Answer from the drawing. Dimensions are ordinates in mm from the lowest x, y and z of the part. A direction names the side the tool comes from. Coordinates: 2 decimals unless noted, no trailing zeros. Write each loop counter-clockwise with the first axis right and the second up, starting at its lowest first coordinate (ties: lowest second). Pieces come first, ordered by that corner, then holes.
1) Find the intervals of material crossed by line 1 (Z direction, x = 1.75, y = 46) (1 decimal); line 2 (Y direction, x = 2, z = 43) (1 decimal); line 3 (Z direction, x = 5, y = 50.5) (1 decimal), in increasing order.
2) Which of the six approach directions +Z, -Z, +X, -X, +Y, -Y give full straight-line access (tool end or side, diameter ignored) to the marked faces 1, 2 and 3?
3) The part is cut by section D-D (z = 38.5). Determine the outline of the cut face in (x, y).
4) Determine the mould class of the marked faces 4, 5, 6 and 7 for opening direction Y: +Y half, -Y half, draft (parallel to the pull), parting line (faces both ways), or undercut.
5) Each of these flat-tipped pins is pushed along its axis until it touches: pin 1 Ø1 at (x, z) = (5.5, 42) entering from -Y; pin 2 Ø5 at (y, z) = (9.94, 45.86) entering from +X; pin 3 Ø3 at (x, y) = (1.5, 44.5) entering from -Z. Where does it stop, or does it pass through?
6) The part is cut by section A-A (y = 7.5). Give the number of separate pieces and of enclosed holes in the cut face, then the cut area to 3 significant figures.
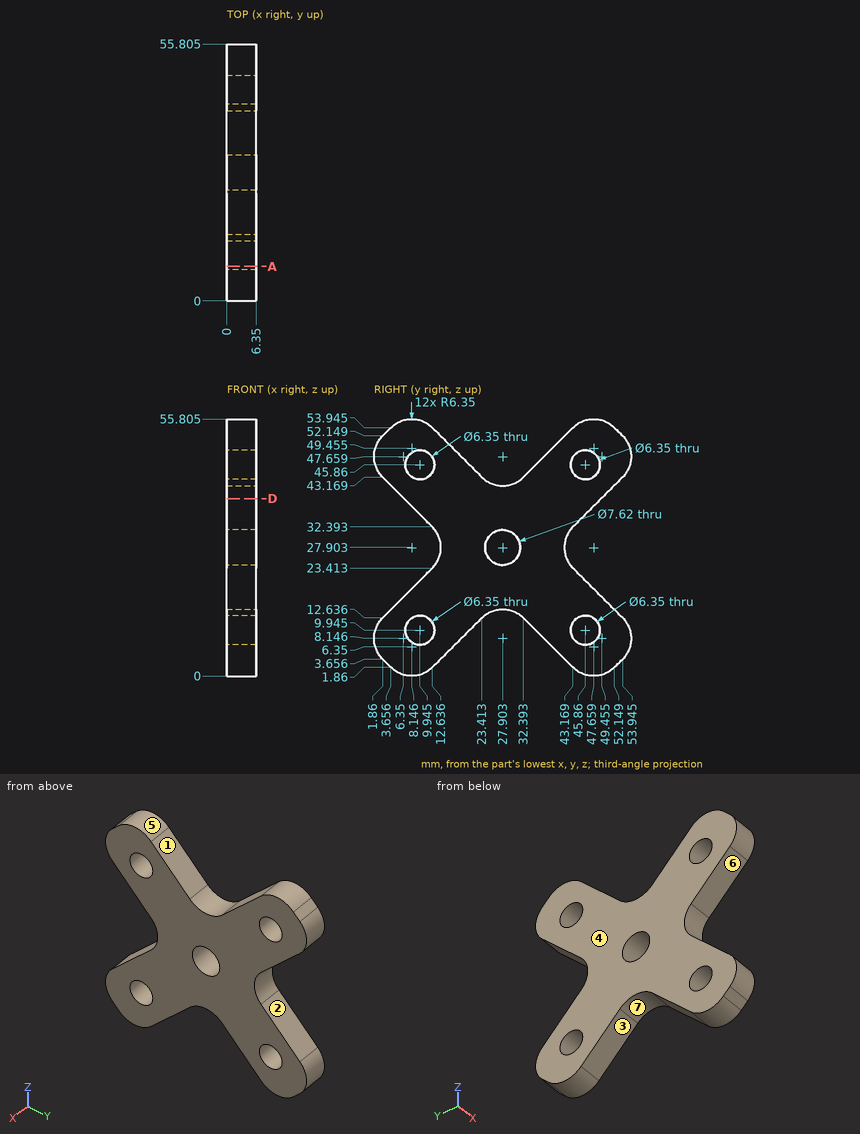
Reported:
1. line 1: z = 0.2 to 6.8, 13.1 to 20.6, 35.2 to 42.7, 49 to 55.6
1. line 2: y = 2 to 8.6, 11.3 to 23.6, 32.2 to 44.5, 47.2 to 53.8
1. line 3: z = 0.7 to 16.1, 39.7 to 55.1
2. face 1: +Z, +X, -X
2. face 2: +X, -X, +Y
2. face 3: -Z, +X, -X
3. outline: (0, 6.53) - (6.35, 6.53) - (6.35, 49.28) - (0, 49.28) - close
4. face 4: draft
4. face 5: undercut
4. face 6: -Y half
4. face 7: undercut
5. pin 1: stops at y = 2.53
5. pin 2: passes through
5. pin 3: stops at z = 0.22
6. separate pieces: 4
6. enclosed holes: 0
6. area: 180 mm2
